from build123d import *

# Parameters (mm, degrees)
F1_DEPTH = 25
F2_DEPTH = 5
F4_DEPTH = 25


with BuildPart() as f1:
    # F0 (on Front) → F1 (new body)
    with BuildSketch(Plane.XZ):
        Polygon((0, 4), (0, 0), (42, 0), (42, 4), (33.5, 4), (25, 4), align=None)
        with BuildLine():
            Line((25, 12.5), (25, 4))
            Line((25, 4), (33.5, 4))
            ThreePointArc((33.5, 4), (27.4895923599, 6.4895923599), (25, 12.5))
        make_face()
        with BuildLine():
            ThreePointArc((25, 12.5), (27.4895923599, 6.4895923599), (33.5, 4))
            ThreePointArc((33.5, 4), (39.5104076401, 6.4895923599), (42, 12.5))
            ThreePointArc((42, 12.5), (33.5, 21), (25, 12.5))
        make_face()
        with BuildLine():
            ThreePointArc((37.5, 12.5), (33.5, 8.5), (29.5, 12.5))
            ThreePointArc((29.5, 12.5), (33.5, 16.5), (37.5, 12.5))
        make_face(mode=Mode.SUBTRACT)
        with BuildLine():
            Line((33.5, 4), (42, 4))
            Line((42, 4), (42, 12.5))
            ThreePointArc((42, 12.5), (39.5104076401, 6.4895923599), (33.5, 4))
        make_face()
    extrude(amount=F1_DEPTH)

    # F0 (on Front) → F2 (join)
    with BuildSketch(Plane.XZ):
        with BuildLine():
            ThreePointArc((37.5, 12.5), (33.5, 16.5), (29.5, 12.5))
            ThreePointArc((29.5, 12.5), (33.5, 8.5), (37.5, 12.5))
        make_face()
    extrude(amount=F2_DEPTH)

    # F3 (on face) → F4 (cut)
    with BuildSketch(Plane.XY.offset(4)):
        with BuildLine():
            ThreePointArc((5, -12.5), (7.5, -15), (10, -12.5))
            Line((10, -12.5), (5, -12.5))
        make_face()
        with BuildLine():
            Line((5, -12.5), (10, -12.5))
            ThreePointArc((10, -12.5), (7.5, -10), (5, -12.5))
        make_face()
        with BuildLine():
            ThreePointArc((15, -12.5), (17.5, -15), (20, -12.5))
            Line((20, -12.5), (15, -12.5))
        make_face()
        with BuildLine():
            Line((15, -12.5), (20, -12.5))
            ThreePointArc((20, -12.5), (17.5, -10), (15, -12.5))
        make_face()
    extrude(amount=-F4_DEPTH, mode=Mode.SUBTRACT)


solid = f1.part
Verification items for the finished model (mm, model axes). A direction names the side the tool comes from. Round coordinates to 2 decimals unless told otherwise and drop trailing zeros. Order: outer loops, then holes, each group sorted by start corner. A loop starts at its lowest first (then second) coordinate and runs counter-clockwise, first axis right, second up. Notation, with made-up numbers: (6, -32.5) -> (32, -32.5) arc R20 ccw to (32, -10.5) -> close; hole circle Ø3 at (31.5, 81.5). An arc over 180 degrees is marked (long way). Put each result on its own line as item: value.
1) Section check B-B (x = 17.5). Record the cut outline in (y, z), then the cut area to 3 significant figures.
Final values:
outline: (-25, 0) -> (-15, 0) -> (-15, 4) -> (-25, 4) -> close; (-10, 0) -> (0, 0) -> (0, 4) -> (-10, 4) -> close
area: 80.0 mm^2
2) Material ranges on line 1 (Z direction, x = 33.5, y = -17); line 2 (X direction, y = -18.5, z = 12.5); line 3 (Y direction, x = 7.5, z = 2), recorded low to high.
Final values:
line 1: z = 0 to 8.5, 16.5 to 21
line 2: x = 25 to 29.5, 37.5 to 42
line 3: y = -25 to -15, -10 to 0
3) Mould release check, pull along X, two halves, no side actions. Record for faces 1 (the flat face through (42, -12, 6)), 2 (the cylindrical face through (15.5, -14, 2)), 3 (the flat face through (0, -12, 2)): +X half, -X half, draft (parallel to the pull), parting line (faces both ways), or undercut.
Final values:
face 1: +X half
face 2: undercut
face 3: -X half
4) Set-up check for faces 4 (the flat face through (13, -12, 4)), 5 (the cylindrical face through (8.65, -14.72, 2.03)), 6 (the flat face through (33, -5, 13)): record each of +Z, -Z, +X, -X, +Y, -Y from which the full face is reachable in a straight line by a thin tool's end or side.
Final values:
face 4: +Z, -X, +Y, -Y
face 5: +Z, -Z
face 6: -Y
5) Section check A-A (y = -12.5). Record the cut outline in (x, z), then the cut area to 3 significant figures.
Final values:
outline: (0, 0) -> (5, 0) -> (5, 4) -> (0, 4) -> close; (10, 0) -> (15, 0) -> (15, 4) -> (10, 4) -> close; (20, 0) -> (42, 0) -> (42, 12.5) arc R8.5 ccw to (25, 12.5) -> (25, 4) -> (20, 4) -> close; hole circle Ø8 at (33.5, 12.5)
area: 336 mm^2
6) Section check C-C (y = -15.75). Record the cut outline in (x, z).
Final values:
outline: (0, 0) -> (42, 0) -> (42, 12.5) arc R8.5 ccw to (25, 12.5) -> (25, 4) -> (0, 4) -> close; hole circle Ø8 at (33.5, 12.5)
7) Depth check by flat-ended pin: pin 1 (7 mm diameter, centred on x = 33.5, z = 12.5, fed in from -Y); pin 2 (5 mm diameter, centred on y = -9, z = 17.5, fed in from +X); pin 3 (1 mm diameter, centred on x = 22.5, y = -15.5, fed in from +Z). Enter the tip coordinate at first touch or a pass-through.
Final values:
pin 1: stops at y = -5
pin 2: stops at x = 41.62
pin 3: stops at z = 4
8) Section check D-D (x = 9.5). Record the cut outline in (y, z), then the cut area to 3 significant figures.
Final values:
outline: (-25, 0) -> (-14, 0) -> (-14, 4) -> (-25, 4) -> close; (-11, 0) -> (0, 0) -> (0, 4) -> (-11, 4) -> close
area: 88.0 mm^2
